```python
from build123d import *

# Parameters (mm, degrees)
FILLET008_R = 2
FILLET013_R = 4


with BuildPart() as part:
    # Cone003 → Cone003 (revolve)
    with BuildSketch(Plane(origin=(7, -12, -84), x_dir=(1, 0, 0), z_dir=(0, -1, 0))):
        Polygon((0, 0), (22, 0), (17, 100), (0, 100), align=None)
    revolve(axis=Axis((7, -12, -84), (0, 0, 1)))

    # Fillet008
    fillet008_edges = [part.edges().sort_by_distance(p)[0] for p in [
        (-15, -12, -84),
    ]]
    fillet(fillet008_edges, radius=FILLET008_R)


with BuildPart() as part_1:
    # Fillet008 placement: moved
    add(part.part.moved(Location((2, -3, 17))))

    # Fillet013
    fillet013_edges = [part_1.edges().sort_by_distance(p)[0] for p in [
        (-8, -15, 33),
    ]]
    fillet(fillet013_edges, radius=FILLET013_R)


solid = part_1.part
```
Geometry check sheet. Reference: the model listing, model coordinates, mm. Coordinates: 2 decimals unless noted, no trailing zeros. Loops run counter-clockwise (first coordinate to the right, second up) from the corner with the lowest first, then second, coordinate; pieces in that order, holes last.
Item 1: Go/stop test with flat-tipped pins: pin 1 Ø1 at (x, z) = (21.5, -15.5) entering from +Y; pin 2 Ø6 at (y, z) = (0, -43) entering from -X; pin 3 Ø1 at (x, z) = (8, 10.5) entering from -Y. Record where each tip stops, or that it passes through.
Item 2: Sectioned sample at A-A, the plane y = -15. Record the boundary of the cut face in (x, z) (1 decimal), then the cut area to 3 significant figures.
Item 3: Sectioned sample at D-D, the plane z = -33. Record the boundary of the cut face in (x, y), then the cut area to 3 significant figures.
Item 4: Sectioned sample at B-B, the plane x = 9. Record the boundary of the cut face in (y, z) (1 decimal), then the cut area to 3 significant figures.
Item 5: Thickness scan on line 1 (Y direction, x = 2.5, z = -1); line 2 (Y direction, x = 12, z = -47.5); line 3 (Z direction, x = -1.5, y = -5.5). Record the ranges inside material, lowest first.
Item 6: Sectioned sample at C-C, the plane z = 16. Record the boundary of the cut face in (x, y), then the cut area to 3 significant figures.
Check result:
1. pin 1: stops at y = 0.28
1. pin 2: stops at x = -8
1. pin 3: stops at y = -33.13
2. outline: (-12.9, -64.9) arc R2 ccw to (-10.9, -67) - (28.9, -67) arc R2 ccw to (30.9, -64.9) - (26.2, 29.2) arc R4 ccw to (22.2, 33) - (-4.2, 33) arc R4 ccw to (-8.2, 29.2) - close
2. area: 3,890 mm2
3. outline: circle Ø40.6 at (9, -15)
3. area: 1,290 mm2
4. outline: (-36.9, -64.9) arc R2 ccw to (-34.9, -67) - (4.9, -67) arc R2 ccw to (6.9, -64.9) - (2.2, 29.2) arc R4 ccw to (-1.8, 33) - (-28.2, 33) arc R4 ccw to (-32.2, 29.2) - close
4. area: 3,890 mm2
5. line 1: y = -32.53 to 2.53
5. line 2: y = -35.81 to 5.81
5. line 3: z = -67 to 32.88
6. outline: circle Ø35.7 at (9, -15)
6. area: 1,000 mm2
